Check sheet for the drawn part. Datum: minimum x, y, z corner. Units: mm. Coordinates: 2 decimals unless noted, no trailing zeros. Write each loop counter-clockwise with the first axis right and the second up, starting at its lowest first coordinate (ties: lowest second). Pieces come first, ordered by that corner, then holes. Notation, with made-up numbers: (52, 30.25) - (86, 30.25) arc R20 cw to (86, 58.25) - close; hole circle Ø8 at (-13, 32.5). An arc over 180 degrees is marked (long way). Use one line per item in the form item = value. Start each with the question number.
1. Cross-section at B-B on z = 9. Record the boundary of the cut face in (x, y), then the cut area to 3 significant figures.
2. Cross-section at C-C on x = 15.75. Record the boundary of the cut face in (y, z).
3. Scan lines: line 1 along X through (y, z) = (11.4, 10); line 2 along Y through (x, z) = (15, 19.45); line 3 along Z through (x, y) = (7.5, 12.1). Record each from-to range of solid material in increasing order.
4. Go/stop test with flat-tipped pins: pin 1 Ø0.9 at (x, y) = (15.5, 6) entering from +Z; pin 2 Ø0.9 at (x, z) = (7, 10) entering from +Y. Record where each tip stops, or that it passes through.
5. Cross-section at A-A on x = 22.5. Record the boundary of the cut face in (y, z).
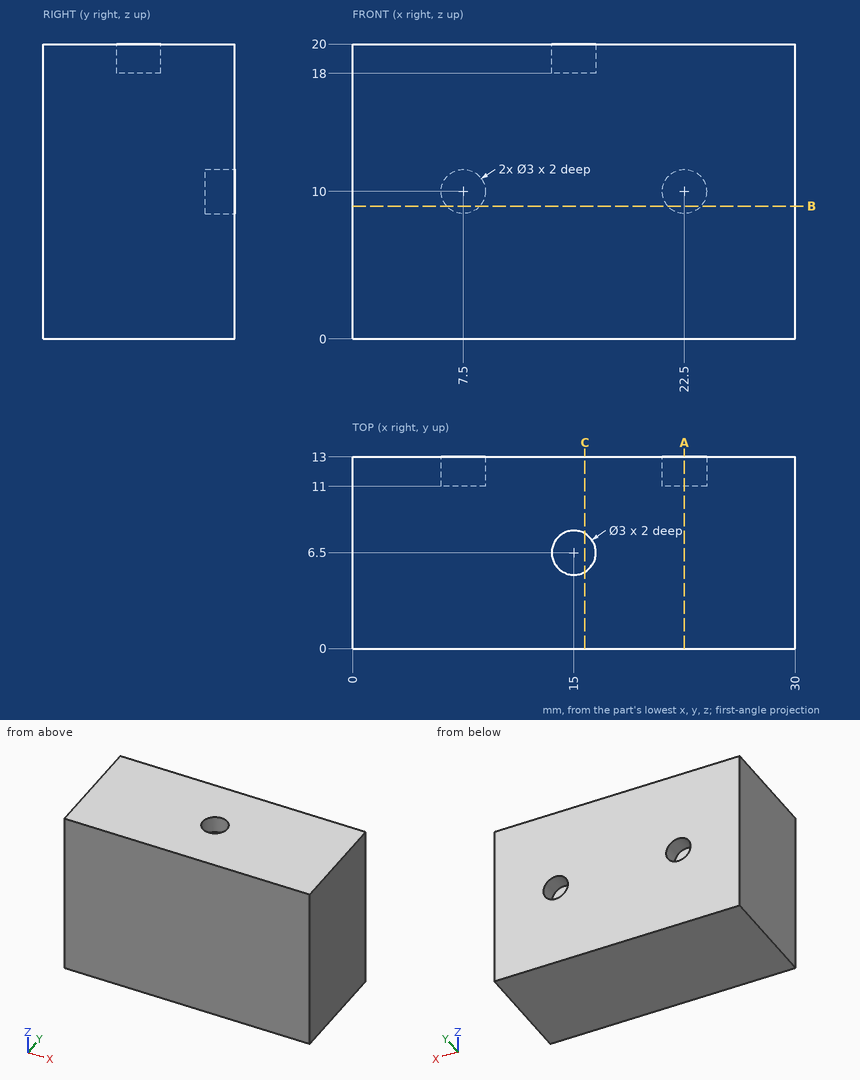
Final values:
q1.outline = (0, 0) - (30, 0) - (30, 13) - (23.62, 13) - (23.62, 11) - (21.38, 11) - (21.38, 13) - (8.62, 13) - (8.62, 11) - (6.38, 11) - (6.38, 13) - (0, 13) - close
q1.area = 381 mm²
q2.outline = (0, 0) - (13, 0) - (13, 20) - (7.8, 20) - (7.8, 18) - (5.2, 18) - (5.2, 20) - (0, 20) - close
q3.line_1 = 0 to 6, 9 to 21, 24 to 30
q3.line_2 = 0 to 5, 8 to 13
q3.line_3 = 0 to 8.5, 11.5 to 20
q4.pin_1 = 18
q4.pin_2 = 11
q5.outline = (0, 0) - (13, 0) - (13, 8.5) - (11, 8.5) - (11, 11.5) - (13, 11.5) - (13, 20) - (0, 20) - close
